Could you check a few things on this drawing? It's one solid part, dimensions in mm from its lowest x, y, z. A direction names the side the tool comes from. Give positions to 0.01 mm unless a question says otherwise; leave off trailing zeros. Order: outer loops, then holes, each group sorted by start corner. A loop starts at its lowest first (then second) coordinate and runs counter-clockwise, first axis right, second up. Notation, with made-up numbers: (-34.75, 15.5) - (-21.75, 15.5) arc R27 ccw to (-21.75, 49.5) - close; hole circle Ø1 at (-37, 24). An arc over 180 degrees is marked (long way). Return JSON: item names as keys, results as strings.
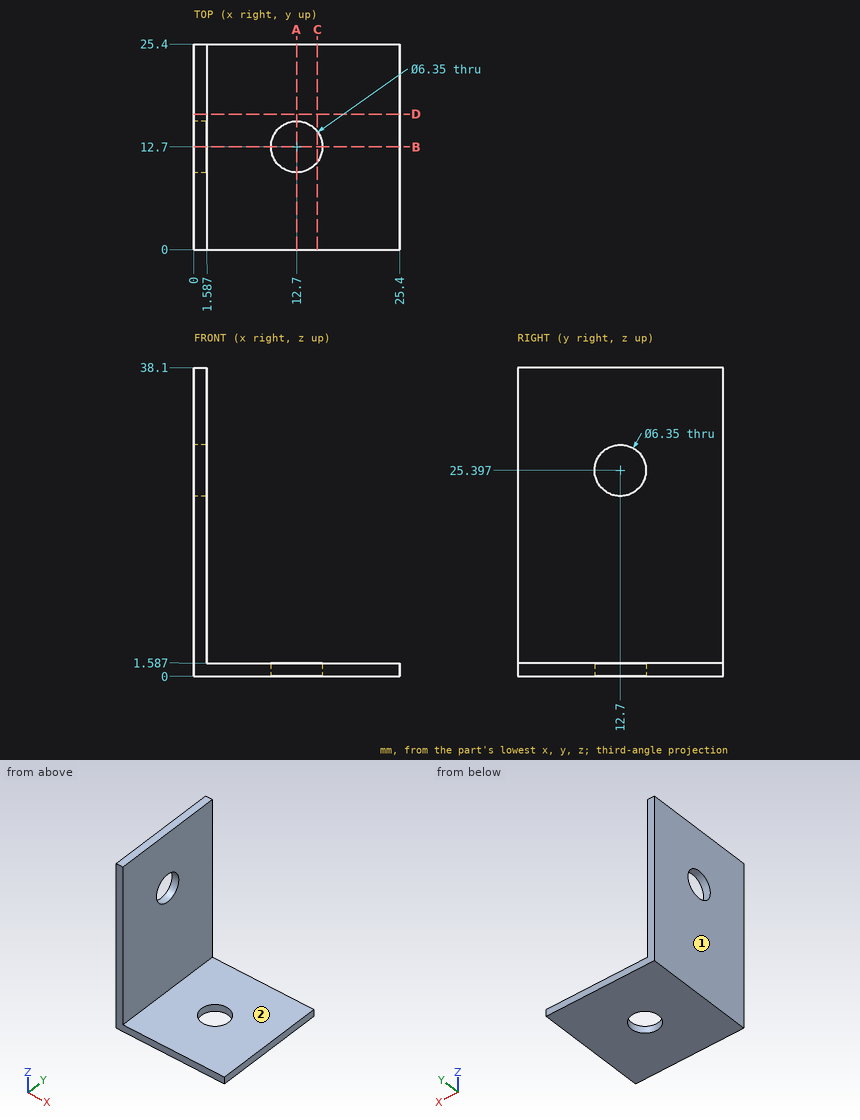
1. Suppose I cut it at B-B (y = 12.7). List the corners of the cut face in (x, z) for me (1 decimal).
Checks:
{"outline": "(0, 0) - (9.5, 0) - (9.5, 1.6) - (1.6, 1.6) - (1.6, 22.2) - (0, 22.2) - close; (0, 28.6) - (1.6, 28.6) - (1.6, 38.1) - (0, 38.1) - close; (15.9, 0) - (25.4, 0) - (25.4, 1.6) - (15.9, 1.6) - close"}
2. Suppose I cut it at A-A (x = 12.7). List the corners of the cut face in (y, z) for me (1 decimal).
Checks:
{"outline": "(0, 0) - (9.5, 0) - (9.5, 1.6) - (0, 1.6) - close; (15.9, 0) - (25.4, 0) - (25.4, 1.6) - (15.9, 1.6) - close"}
3. For pin 1 Ø7.5 at (y, z) = (8.5, 14) entering from +X; pin 2 Ø10 at (x, y) = (12.7, 12.7) entering from +Z, each with a flat end and sliding along its axis, tell me the tip position at first contact or that it passes through.
Checks:
{"pin 1": "x = 1.59", "pin 2": "z = 1.59"}
4. On a 3-axis mill with a long thin cutter (end or side, diameter ignored), from which of +Z, -Z, +X, -X, +Y, -Y can I reach the whole of each face in a straight line? I mean the marked faces 1 and 2. Say none if no direction works.
Checks:
{"face 1": "+Z, -Z, -X, +Y, -Y", "face 2": "+Z, +X, +Y, -Y"}
5. Suppose I cut it at C-C (x = 15.25). List the corners of the cut face in (y, z) for me.
Checks:
{"outline": "(0, 0) - (10.81, 0) - (10.81, 1.59) - (0, 1.59) - close; (14.59, 0) - (25.4, 0) - (25.4, 1.59) - (14.59, 1.59) - close"}
6. If I drill on L1, parallel to Z at x = 0.45, y = 12.7; L2, parallel to X at y = 9.75, z = 16, over which ranges is the centre line in solid material (lowest first)? Write a range as [from, to].
Checks:
{"L1": "[0, 22.22], [28.57, 38.1]", "L2": "[0, 1.59]"}
7. Suppose I cut it at D-D (y = 16.75). List the corners of the cut face in (x, z) for me.
Checks:
{"outline": "(0, 0) - (25.4, 0) - (25.4, 1.59) - (1.59, 1.59) - (1.59, 38.1) - (0, 38.1) - close"}
